```python
from build123d import *

# Parameters (mm, degrees)
SKETCH1_W           = 635
SKETCH1_H           = 25.4
BOSS_EXTRUDE1_DEPTH = 50.8
SKETCH2_R           = 5.08
CUT_EXTRUDE1_DEPTH  = 53.34
SKETCH3_W           = 635
SKETCH3_H           = 40.64
CUT_EXTRUDE2_DEPTH  = 22.098


with BuildPart() as part:
    # Sketch1 → Boss-Extrude1 (new body)
    with BuildSketch(Plane(origin=(0, 0, 0), x_dir=(1, 0, 0), z_dir=(0, 1, 0))):
        Rectangle(SKETCH1_W, SKETCH1_H)
    extrude(amount=BOSS_EXTRUDE1_DEPTH)

    # Sketch2 → Cut-Extrude1 (cut)
    with BuildSketch(Plane(origin=(0, 50.8, 0), x_dir=(1, 0, 0), z_dir=(0, 1, 0))):
        with Locations(Location((-300.99, 0, 0), (0, 0, 270))):
            Circle(SKETCH2_R)
        with Locations(Location((-287.02, 0, 0), (0, 0, 270))):
            Circle(SKETCH2_R)
        with Locations(Location((300.99, 0, 0), (0, 0, 270))):
            Circle(SKETCH2_R)
        with Locations(Location((287.02, 0, 0), (0, 0, 270))):
            Circle(SKETCH2_R)
    extrude(amount=-CUT_EXTRUDE1_DEPTH, mode=Mode.SUBTRACT)

    # Sketch3 → Cut-Extrude2 (cut)
    with BuildSketch(Plane.XY.offset(12.7)):
        with Locations((0, 25.4)):
            Rectangle(SKETCH3_W, SKETCH3_H)
    extrude(amount=-CUT_EXTRUDE2_DEPTH, mode=Mode.SUBTRACT)


solid = part.part
```
Read the model definition and answer for the solid it produces. Units are mm, in the model's axes. A direction names the side the tool comes from. Give positions to 0.01 mm unless a question says otherwise; leave off trailing zeros. Loops run counter-clockwise (first coordinate to the right, second up) from the corner with the lowest first, then second, coordinate; pieces in that order, holes last.
Item 1: The mould has two halves that part along X. Classify faces 3 (the flat face through (-4, 50.8, 0)), 4 (the cylindrical face through (-296.707, 2.576, 2.731)), 5 (the cylindrical face through (296.03, 2.58, -1.1)), 6 (the flat face through (-317.5, 27, -10)): released by +X, released by -X, zero draft, split by the parting line, or undercut.
Item 2: The part is cut by section A-A (x = 19.5). Write down the section's boundary in (y, z), and give its area (3 significant figures).
Item 3: The part is cut by section C-C (y = 39). Write down the section's boundary in (x, z), and give its area (3 significant figures).
Item 4: The part is cut by section B-B (z = 0). Give the number of separate pieces and of enclosed holes in the cut face, and give its area (3 significant figures).
Item 5: For faces 1 (the flat face through (-4, 26, -9.398)), 2 (the cylindrical face through (-281.983, 48.296, -0.661)), determine the directions among +Z, -Z, +X, -X, +Y, -Y from which every point of the face is accessible in a straight line to the end or side of a thin tool.
Item 6: Each of these flat-tipped pins is pushed along its axis until it touches: pin 1 Ø11.5 at (x, z) = (-300.99, 0) entering from +Y; pin 2 Ø20.5 at (x, y) = (-72, 15.5) entering from +Z. Where does it stop, or does it pass through?
Item 7: Find the intervals of material crossed by line 1 along X through (y, z) = (49.2, 0); line 2 along Z through (x, y) = (300.99, 47.3); line 3 along Y through (x, z) = (-256, 0.5), in increasing order.
Taken from the geometry:
1. face 3: zero draft
1. face 4: undercut
1. face 5: undercut
1. face 6: released by -X
2. outline: (0, -12.7) - (50.8, -12.7) - (50.8, 12.7) - (45.72, 12.7) - (45.72, -9.4) - (5.08, -9.4) - (5.08, 12.7) - (0, 12.7) - close
2. area: 392 mm2
3. outline: (-317.5, -12.7) - (317.5, -12.7) - (317.5, -9.4) - (-317.5, -9.4) - close
3. area: 2,100 mm2
4. separate pieces: 10
4. enclosed holes: 0
4. area: 6,040 mm2
5. face 1: +Z, +X, -X
5. face 2: +Y, -Y
6. pin 1: stops at y = 50.8
6. pin 2: stops at z = -9.4
7. line 1: x = -317.5 to -306.07, -295.91 to -292.1, -281.94 to 281.94, 292.1 to 295.91, 306.07 to 317.5
7. line 2: z = -12.7 to -5.08, 5.08 to 12.7
7. line 3: y = 0 to 5.08, 45.72 to 50.8
